from build123d import *

# Parameters (mm, degrees)
SKETCH1_W           = 77
SKETCH1_H           = 80
SKETCH1_R           = 3
SKETCH1_W_2         = 40
SKETCH1_H_2         = 25
BOSS_EXTRUDE1_DEPTH = 4
CUT_EXTRUDE1_DEPTH  = 10
SKETCH3_R           = 35.5
SKETCH3_R_2         = 32
BOSS_EXTRUDE2_DEPTH = 110
SKETCH5_R           = 32
BOSS_EXTRUDE3_DEPTH = 5


with BuildPart() as part:
    # Sketch1 → Boss-Extrude1 (new, symmetric)
    with BuildSketch(Plane(origin=(0, 0, 0), x_dir=(1, 0, 0), z_dir=(0, 1, 0))):
        Rectangle(SKETCH1_W, SKETCH1_H)
        with Locations(Location((-28.501375206, 30, 0), (0, 0, 270))):
            Circle(SKETCH1_R, mode=Mode.SUBTRACT)
        with Locations(Location((28.5, 30, 0), (0, 0, 270))):
            Circle(SKETCH1_R, mode=Mode.SUBTRACT)
        with Locations(Location((28.5, -30, 0), (0, 0, 90))):
            Circle(SKETCH1_R, mode=Mode.SUBTRACT)
        with Locations(Location((-28.501375206, -30, 0), (0, 0, 90))):
            Circle(SKETCH1_R, mode=Mode.SUBTRACT)
        Rectangle(SKETCH1_W_2, SKETCH1_H_2, mode=Mode.SUBTRACT)
    extrude(amount=BOSS_EXTRUDE1_DEPTH, both=True)

    # Sketch2 → Cut-Extrude1 (cut)
    with BuildSketch(Plane(origin=(0, 0, 0), x_dir=(1, 0, 0), z_dir=(0, 1, 0))):
        Polygon((-33.501375206, -32.886751346), (-33.501375206, -27.113248654), (-28.501375206, -24.226497308), (-23.501375206, -27.113248654), (-23.501375206, -30), (-23.501375206, -32.886751346), (-28.501375206, -35.773502692), align=None)
        Polygon((-23.501375206, 30), (-23.501375206, 27.113248654), (-28.501375206, 24.226497308), (-33.501375206, 27.113248654), (-33.501375206, 32.886751346), (-28.501375206, 35.773502692), (-23.501375206, 32.886751346), align=None)
        Polygon((23.501375206, -30), (23.501375206, -27.113248654), (28.501375206, -24.226497308), (33.501375206, -27.113248654), (33.501375206, -32.886751346), (28.501375206, -35.773502692), (23.501375206, -32.886751346), align=None)
        Polygon((23.501375206, 27.113248654), (28.501375206, 24.226497308), (33.501375206, 27.113248654), (33.501375206, 32.886751346), (28.501375206, 35.773502692), (23.501375206, 32.886751346), (23.501375206, 30), align=None)
    extrude(amount=CUT_EXTRUDE1_DEPTH, mode=Mode.SUBTRACT)

    # Sketch3 → Boss-Extrude2 (add)
    with BuildSketch(Plane(origin=(0, 0, 0), x_dir=(1, 0, 0), z_dir=(0, 1, 0))):
        with Locations(Location((0, 0, 0), (0, 0, 270))):
            Circle(SKETCH3_R)
        with Locations(Location((0, 0, 0), (0, 0, 270))):
            Circle(SKETCH3_R_2, mode=Mode.SUBTRACT)
    extrude(amount=BOSS_EXTRUDE2_DEPTH)

    # Sketch5 → Boss-Extrude3 (add, symmetric)
    with BuildSketch(Plane(origin=(0, 4, 0), x_dir=(1, 0, 0), z_dir=(0, 1, 0))):
        with Locations(Location((0, 0, 0), (0, 0, 270))):
            Circle(SKETCH5_R)
    extrude(amount=BOSS_EXTRUDE3_DEPTH, both=True)


solid = part.part
The model under review builds one solid part; all positions refer to its coordinate system, in mm. A direction names the side the tool comes from. Coordinates: 2 decimals unless noted, no trailing zeros. Write each loop counter-clockwise with the first axis right and the second up, starting at its lowest first coordinate (ties: lowest second). Pieces come first, ordered by that corner, then holes. Notation, with made-up numbers: (-4, -8.75) - (26, -8.75) arc R28 ccw to (26, 17.25) - close; hole circle Ø6 at (64.25, 60). An arc over 180 degrees is marked (long way). Answer as a JSON object with one key per item and string values. Group by question number.
1. Machinability: for faces 4 (the face through (-1, 0, -40)), 5 (the face through (0, 9, 0)), 6 (the face through (0, -1, 0)), which of the approach directions +Z, -Z, +X, -X, +Y, -Y give a long, thin tool a straight path to every point of the face, cutting with its end or side? Answer none if there is none.
2. Clearance check with flat-ended pins moving along their axes: pin 1 Ø5 at (y, z) = (91.5, -28) entering from -X; pin 2 Ø3 at (x, z) = (-30, -27.5) entering from +Y; pin 3 Ø8 at (x, z) = (30.5, -31.5) entering from +Y. State where each tip first meets the part, or that it passes through.
3. Add section A-A (z = 0). Give the boundary of the cut face in (x, y), plus the area to 3 significant figures.
4. Add section C-C (z = -30). Give the boundary of the cut face in (x, y), plus the area to 3 significant figures.
5. To check wall thickness, follow probe 1 along X at (y, z) = (-2.1, 30); probe 2 along Z at (x, y) = (28.5, -2.8); probe 3 along Y at (x, z) = (-29.5, -35). State the ranges of each line that lie inside material, in increasing order.
6. Add section B-B (x = 0). Give the boundary of the cut face in (y, z).
7. Add section D-D (y = 100). Give the boundary of the cut face in (x, z).
8. Mouldability with a two-part tool opening along Z and no side actions: class faces 1 (the face through (30.97, 1.97, 25.65)), 2 (the face through (38.5, 0, 1)), 3 (the face through (-31.495, 56.258, 16.381)) as pulls with the +Z half, pulls with the -Z half, needs draft (parallel to the pull), parting line crosses it, or undercut.
Findings:
{
 "1": {"face 4": "-Z, +X, -X, +Y, -Y", "face 5": "+Y", "face 6": "-Y"},
 "2": {"pin 1": "x = -24.7", "pin 2": "y = 0", "pin 3": "y = 4"},
 "3": {"outline": "(-38.5, -4) - (-20, -4) - (-20, -1) - (20, -1) - (20, -4) - (38.5, -4) - (38.5, 4) - (35.5, 4) - (35.5, 110) - (32, 110) - (32, 9) - (-32, 9) - (-32, 110) - (-35.5, 110) - (-35.5, 4) - (-38.5, 4) - close", "area": "1,560 mm²"},
 "4": {"outline": "(-38.5, -4) - (-31.5, -4) - (-31.5, 0) - (-33.5, 0) - (-33.5, 4) - (-38.5, 4) - close; (-25.5, -4) - (25.5, -4) - (25.5, 0) - (23.5, 0) - (23.5, 4) - (18.98, 4) - (18.98, 110) - (11.14, 110) - (11.14, 9) - (-11.14, 9) - (-11.14, 110) - (-18.98, 110) - (-18.98, 4) - (-23.5, 4) - (-23.5, 0) - (-25.5, 0) - close; (31.5, -4) - (38.5, -4) - (38.5, 4) - (33.5, 4) - (33.5, 0) - (31.5, 0) - close", "area": "2,260 mm²"},
 "5": {"probe 1": "-38.5 to -31.5, -25.5 to 25.5, 31.5 to 38.5", "probe 2": "-40 to -33, -27 to 27, 33 to 40", "probe 3": "-4 to 0"},
 "6": {"outline": "(-4, -40) - (4, -40) - (4, -35.5) - (110, -35.5) - (110, -32) - (9, -32) - (9, 32) - (110, 32) - (110, 35.5) - (4, 35.5) - (4, 40) - (-4, 40) - (-4, 12.5) - (-1, 12.5) - (-1, -12.5) - (-4, -12.5) - close"},
 "7": {"outline": "circle Ø71 at (0, 0); hole circle Ø64 at (0, 0)"},
 "8": {"face 1": "undercut", "face 2": "needs draft", "face 3": "parting line crosses it"}
}
